Autodesk Inventor part; units mm, degrees
ref_plane "YZ Plane" through (0, 0, 0) normal (1, 0, 0) x (0, 1, 0)
ref_plane "XZ Plane" through (0, 0, 0) normal (0, 1, 0) x (-1, 0, 0)
ref_plane "XY Plane" through (0, 0, 0) normal (0, 0, 1) x (1, 0, 0)
sketch "Sketch1" plane through (0, 0, 0) normal (0, 0, 1) x (1, 0, 0)
  line L0 (0, 0) -> (0, 8)
  line L1 (0, 8) -> (4, 8)
  line L2 (4, 8) -> (8, 4)
  line L3 (8, 4) -> (18, 4)
  line L4 (18, 4) -> (18, 0)
  line L5 (18, 0) -> (0, 0)
  dimension "d0" = 18
  dimension "d1" = 4
  dimension "d2" = 8
  dimension "d3" = 4
  dimension "d4" = 45
extrude "Extrusion1" add sketch "Sketch1" along normal blind 4
sketch "Sketch2" plane through (0, 0, 0) normal (-1, 0, 0) x (0, 0, 1)
  line L0 (0, 0) -> (0, 8)
  line L1 (0, 0) -> (4, 0)
  line L2 (4, 8) -> (4, 0)
  line L3 (0, 8) -> (4, 8)
  line L4 (2, 0) -> (2, 8) construction
  line L5 (0, 4) -> (4, 4) construction
  point P0 (2, 2)
  point P1 (2, 6)
  dimension "d7" = 4
hole "Hole1" at (0, 2, 2) at (0, 6, 2) direction (1, 0, 0) diameter 1.6 depth 5 tip angle 118
sketch "Sketch3" plane through (18, 0, 0) normal (1, 0, 0) x (0, 0, -1)
  line L0 (0, 4) -> (0, 0)
  line L1 (0, 4) -> (-4, 4)
  line L2 (-4, 0) -> (-4, 4)
  line L3 (0, 0) -> (-4, 0)
  line L4 (0, 0) -> (-4, 4) construction
  point P0 (0, 0)
  point P1 (-2, 2)
hole "Hole2" at (18, 2, 2) direction (-1, 0, 0) diameter 1.6 depth 5 tip angle 118
properties part number "support 1"
Can you work these out from the model? Positions are in its coordinate system, mm. A direction names the side the tool comes from. Give positions to 0.01 mm unless a question says otherwise; leave off trailing zeros. Write each loop counter-clockwise with the first axis right and the second up, starting at its lowest first coordinate (ties: lowest second). Pieces come first, ordered by that corner, then holes. Notation, with made-up numbers: (-1, 23) -> (14, 23) arc R16 cw to (14, 40) -> close; hole circle Ø11 at (3, 86.5). An arc over 180 degrees is marked (long way). Answer as a JSON object with one key per item and string values. Group by question number.
Item 1: I'm going to push flat-ended pins straight in: P1, Ø2, axis at y = 6, z = 1, coming from the +X side; P2, Ø1.8, axis at y = 6, z = 2, coming from the +X side. Where does each tip first touch, or does it pass through?
Item 2: Suppose I cut it at B-B (z = 3.45). Please give me the cut outline in (x, y).
Item 3: For faces 4 (the face through (7, 3, 4)), 5 (the face through (18, 3, 2)), 6 (the face through (13, 4, 2)), 7 (the face through (2.54, 6.71, 2.37)), 8 (the face through (15.46, 1.46, 2.59)), which set-ups out of +Z, -Z, +X, -X, +Y, -Y let a thin tool reach every point of the face, with its end or its side?
Item 4: Suppose I cut it at A-A (x = 2.25). Please give me the cut outline in (y, z).
Item 5: Suppose I cut it at C-C (x = 15.5). Please give me the cut outline in (y, z), plus the area to 3 significant figures.
Item 6: Please list where these lines run through material, in increasing order: line 1 (Y direction, x = 2.6, z = 2); line 2 (Z direction, x = 2.45, y = 6); line 3 (Y direction, x = 2.25, z = 2.35). Write a range as [from, to].
Item 7: Suppose I cut it at D-D (y = 4.25). Please give me the cut outline in (x, z).
Item 8: We'd pull the mould along Y, two halves only. Please class faces 1 (the face through (0, 4, 2)), 2 (the face through (2, 8, 2)), 3 (the face through (2.535, 1.325, 2.43)): +Y half, -Y half, draft (parallel to the pull), parting line (faces both ways), or undercut.
Findings:
{
 "1": {"P1": "stops at x = 7", "P2": "stops at x = 6.9"},
 "2": {"outline": "(0, 0) -> (18, 0) -> (18, 4) -> (8, 4) -> (4, 8) -> (0, 8) -> close"},
 "3": {"face 4": "+Z, +X, -X, +Y, -Y", "face 5": "+Z, -Z, +X, +Y, -Y", "face 6": "+Z, -Z, +X, +Y", "face 7": "-X", "face 8": "+X"},
 "4": {"outline": "(0, 0) -> (8, 0) -> (8, 4) -> (0, 4) -> close; hole circle Ø1.6 at (2, 2); hole circle Ø1.6 at (6, 2)"},
 "5": {"outline": "(0, 0) -> (4, 0) -> (4, 4) -> (0, 4) -> close; hole circle Ø1.6 at (2, 2)", "area": "14.0 mm²"},
 "6": {"line 1": "y = [0, 1.2], [2.8, 5.2], [6.8, 8]", "line 2": "z = [0, 1.2], [2.8, 4]", "line 3": "y = [0, 1.28], [2.72, 5.28], [6.72, 8]"},
 "7": {"outline": "(0, 0) -> (7.75, 0) -> (7.75, 4) -> (0, 4) -> close"},
 "8": {"face 1": "draft", "face 2": "+Y half", "face 3": "undercut"}
}
